Design review of the part built by this model. Coordinates are the model's own, in mm. A direction names the side the tool comes from. Coordinates: 2 decimals unless noted, no trailing zeros. Order: outer loops, then holes, each group sorted by start corner. A loop starts at its lowest first (then second) coordinate and runs counter-clockwise, first axis right, second up. Notation, with made-up numbers: M 51.25,44 L 58.25,44 A21 ccw 58.25,72 Z; hole C -12.5,7 d8. An arc over 180 degrees is marked long. Answer in a Markdown table with one row per item.
from build123d import *

# Parameters (mm, degrees)
F0_W     = 179
F0_H     = 109
F0_R     = 1.75
F0_R_2   = 4
F1_DEPTH = 2.4
F2_DEPTH = 20.5
F3_R     = 0.4


with BuildPart() as f1:
    # F0 (on Top) → F1 (new body)
    with BuildSketch(Plane.XY):
        with Locations((-1, -0.096982)):
            Rectangle(F0_W, F0_H)
        with Locations((-87, -51.096982)):
            Circle(F0_R, mode=Mode.SUBTRACT)
        with Locations((-12.5, -34.596982)):
            Circle(F0_R_2, mode=Mode.SUBTRACT)
        with Locations((85, -51.096982)):
            Circle(F0_R, mode=Mode.SUBTRACT)
        with Locations((39.5, -26.596982)):
            Circle(F0_R_2, mode=Mode.SUBTRACT)
        with Locations((-48, -0.096982)):
            Circle(F0_R, mode=Mode.SUBTRACT)
        with Locations((-12.5, 25.403018)):
            Circle(F0_R_2, mode=Mode.SUBTRACT)
        with Locations((-87, 50.903018)):
            Circle(F0_R, mode=Mode.SUBTRACT)
        with Locations((39.5, 25.403018)):
            Circle(F0_R_2, mode=Mode.SUBTRACT)
        with Locations((65, -0.096982)):
            Circle(F0_R, mode=Mode.SUBTRACT)
        with Locations((0, 50.903018)):
            Circle(F0_R, mode=Mode.SUBTRACT)
        with Locations((85, 50.903018)):
            Circle(F0_R, mode=Mode.SUBTRACT)
        with Locations((-12.5, 25.403018)):
            Circle(F0_R_2)
        with Locations((39.5, 25.403018)):
            Circle(F0_R_2)
        with Locations((-12.5, -34.596982)):
            Circle(F0_R_2)
        with Locations((39.5, -26.596982)):
            Circle(F0_R_2)
    extrude(amount=-F1_DEPTH)

    # F0 (on Top) → F2 (join)
    with BuildSketch(Plane.XY):
        with Locations((-12.5, 25.403018)):
            Circle(F0_R_2)
        with Locations((-12.5, -34.596982)):
            Circle(F0_R_2)
        with Locations((39.5, -26.596982)):
            Circle(F0_R_2)
        with Locations((39.5, 25.403018)):
            Circle(F0_R_2)
    extrude(amount=F2_DEPTH)

    # F3
    f3_edges = [f1.edges().sort_by_distance(p)[0] for p in [
        (-1, 54.403018, -2.4),
        (-90.5, -0.096982, -2.4),
        (88.5, -0.096982, -2.4),
        (-1, -54.596982, -2.4),
    ]]
    fillet(f3_edges, radius=F3_R)


solid = f1.part
(1) Draft analysis for pull direction X (two halves, no side actions). For faces 3 (the flat face through (-13, 25, 20.5)), 4 (the cylindrical face through (86.617, 50.233, -1.183)), 5 (the cylindrical face through (-86.19, -52.65, -1.18)), state which applies: pulls with the +X half, pulls with the -X half, needs draft (parallel to the pull), parting line crosses it, or undercut.
Return value:
| item | result |
|---|---|
| face 3 | needs draft |
| face 4 | undercut |
| face 5 | undercut |
(2) For faces 1 (the cylindrical face through (-46.383, -0.767, -1.183)), 2 (the cylindrical face through (36.3, -29, 10.1)), list the 3-axis set-ups (+Z, -Z, +X, -X, +Y, -Y) from which the entire face can be reached by the end or side of a thin tool; tool diameter is ignored.
Return value:
| item | result |
|---|---|
| face 1 | +Z, -Z |
| face 2 | +Z |
(3) Add section B-B, the plane y = -5. Give the boundary of the cut face in (x, z), and give its area (3 significant figures).
Return value:
| item | result |
|---|---|
| outline | M -90.5,-2 A0.4 ccw -90.1,-2.4 L 88.1,-2.4 A0.4 ccw 88.5,-2 L 88.5,0 L -90.5,0 Z |
| area | 430 mm2 |
(4) Add section A-A, the plane x = -87. Give the boundary of the cut face in (y, z), and give its area (3 significant figures).
Return value:
| item | result |
|---|---|
| outline | M -54.6,-2 A0.4 ccw -54.2,-2.4 L -52.85,-2.4 L -52.85,0 L -54.6,0 Z; M -49.35,-2.4 L 49.15,-2.4 L 49.15,0 L -49.35,0 Z; M 52.65,-2.4 L 54,-2.4 A0.4 ccw 54.4,-2 L 54.4,0 L 52.65,0 Z |
| area | 245 mm2 |
(5) Add section C-C, the plane z = 8. Give the boundary of the cut face in (x, y).
Return value:
| item | result |
|---|---|
| outline | C -12.5,-34.6 d8; C -12.5,25.4 d8; C 39.5,-26.6 d8; C 39.5,25.4 d8 |
(6) For line 1 along Y through (x, z) = (85, -0.65); line 2 along Y through (x, z) = (-48, -0.65); line 3 along Z through (x, y) = (-28, -21.5), list the stretches that pass through material, from the lowest coordinate up. Write a range as from..to.
Return value:
| item | result |
|---|---|
| line 1 | y = -54.6..-52.85, -49.35..49.15, 52.65..54.4 |
| line 2 | y = -54.6..-1.85, 1.65..54.4 |
| line 3 | z = -2.4..0 |
(7) Insertion check: pin 1 Ø4.5 at (x, y) = (65, -0.1) entering from +Z; pin 2 Ø4 at (x, z) = (-19.5, 12.5) entering from -Y; pin 3 Ø8 at (x, z) = (-16.5, 17) entering from -Y; pin 4 Ø8 at (x, z) = (36, 6.5) entering from -Y. Each pin has a flat end and moves straight along its axis. Give the tip position at first contact, or say it passes through.
Return value:
| item | result |
|---|---|
| pin 1 | stops at z = 0 |
| pin 2 | passes through |
| pin 3 | stops at y = -38.6 |
| pin 4 | stops at y = -30.6 |
(8) Add section D-D, the plane x = 11.5. Give the boundary of the cut face in (y, z).
Return value:
| item | result |
|---|---|
| outline | M -54.6,-2 A0.4 ccw -54.2,-2.4 L 54,-2.4 A0.4 ccw 54.4,-2 L 54.4,0 L -54.6,0 Z |
